Autodesk Inventor part; units mm, degrees
ref_plane "YZ Plane" through (0, 0, 0) normal (1, 0, 0) x (0, 1, 0)
ref_plane "XZ Plane" through (0, 0, 0) normal (0, 1, 0) x (-1, 0, 0)
ref_plane "XY Plane" through (0, 0, 0) normal (0, 0, 1) x (1, 0, 0)
sketch "Sketch1" plane through (0, 0, 0) normal (0, 0, 1) x (1, 0, 0)
  line L0 (58.4, 13.1) -> (-58.4, 13.1)
  line L1 (-58.4, 13.1) -> (-58.4, -13.1)
  line L2 (-58.4, -13.1) -> (58.4, -13.1)
  line L3 (58.4, -13.1) -> (58.4, 13.1)
  line L4 (58.4, 13.1) -> (-58.4, -13.1) construction
  line L5 (-58.4, 13.1) -> (58.4, -13.1) construction
  point P0 (0, 0)
  dimension "d0" = 116.8
  dimension "d1" = 26.2
extrude "Extrusion1" add sketch "Sketch1" along normal blind 11
sketch "Sketch2" plane through (58.4, -13.1, 0) normal (1, 0, 0) x (0, 0, -1)
  line L0 (0, 0) -> (0, 26.2)
  line L1 (0, 26.2) -> (-11, 26.2)
  line L2 (-11, 0) -> (-11, 26.2)
  line L3 (0, 0) -> (-11, 0)
  line L4 (-11, 26.2) -> (-11, 0)
  line L5 (-11, 26.2) -> (-5, 26.2)
  line L6 (-5, 26.2) -> (-5, 23.2)
  line L7 (-5, 23.2) -> (-11, 23.2)
  line L8 (-11, 23.2) -> (-11, 26.2)
  line L9 (-11, 23.2) -> (-8.4, 23.2)
  line L10 (-8.4, 23.2) -> (-8.4, 20.2)
  line L11 (-8.4, 20.2) -> (-11, 20.2)
  line L12 (-11, 20.2) -> (-11, 23.2)
  line L13 (-11, 26.2) -> (-5, 26.2)
  line L14 (-5, 26.2) -> (-5, 10.1)
  line L15 (-5, 10.1) -> (-11, 10.1)
  line L16 (-11, 10.1) -> (-11, 26.2)
  line L17 (-11, 10.1) -> (-5, 10.1)
  line L18 (-5, 10.1) -> (-5, 13.1)
  line L19 (-5, 13.1) -> (-11, 13.1)
  line L20 (-11, 13.1) -> (-11, 10.1)
  line L21 (-11, 13.1) -> (-8.4, 13.1)
  line L22 (-8.4, 13.1) -> (-8.4, 16.1)
  line L23 (-8.4, 16.1) -> (-11, 16.1)
  line L24 (-11, 16.1) -> (-11, 13.1)
  point P0 (0, 13.1)
  point P1 (-11, 16.1)
  point P2 (-11, 20.2)
  dimension "d4" = 6
  dimension "d5" = 3
  dimension "d6" = 2.6
  dimension "d7" = 3
  dimension "d8" = 16.1
  dimension "d9" = 3
  dimension "d10" = 2.6
  dimension "d11" = 3
extrude "Extrusion2" cut sketch "Sketch2" against normal blind 113.8 contours L14 L19 L22 L23 L2 L11 L10 L7
fillet "Fillet1" radius 2 5 edges at (58.4, 10.1, 11) (58.4, -5.05, 11) (-58.4, 0, 11) (58.4, 0, 0) (-58.4, 0, 0)
sketch "Sketch4" plane through (-56.4, -13.1, 0) normal (0, -1, 0) x (1, 0, 0)
  arc A0 (-2, 2) -> (0, 0) centre (0, 2) ccw
  line L0 (0, 0) -> (112.8, 0)
  arc A1 (112.8, 0) -> (114.8, 2) centre (112.8, 2) ccw
  line L1 (114.8, 2) -> (114.8, 9)
  arc A2 (114.8, 9) -> (112.8, 11) centre (112.8, 9) ccw
  line L2 (0, 11) -> (112.8, 11)
  arc A3 (0, 11) -> (-2, 9) centre (0, 9) ccw
  line L3 (-2, 2) -> (-2, 9)
  circle A4 centre (104.8, 5.5) radius 4.1
  circle A5 centre (97.8, 5.5) radius 2.15
  line L4 (97.8, 7.65) -> (101.3089, 7.65)
  line L5 (97.8, 3.35) -> (101.3089, 3.35)
  circle A6 centre (15, 5.5) radius 4.1
  circle A7 centre (8, 5.5) radius 2.15
  line L6 (8, 3.35) -> (11.5089, 3.35)
  line L7 (8, 7.65) -> (11.5089, 7.65)
  point P0 (56.4, 0)
  point P1 (114.8, 5.5)
  point P2 (12.2407, 8.5325)
  point P3 (8.4381, 3.3951)
  point P4 (11.1965, 3.9692)
  point P5 (-2, 5.5)
  dimension "d19" = 8.2
  dimension "d20" = 4.3
  dimension "d21" = 7
  dimension "d22" = 0
  dimension "d23" = 10
  dimension "d24" = 8.2
  dimension "d25" = 4.3
  dimension "d26" = 7
  dimension "d27" = 10
  dimension "d28" = 0
  dimension "d40" = 0
extrude "Extrusion4" cut sketch "Sketch4" against normal blind 5.2 contours A4 | A4 L5 A5 L4 | A5 | A6 | A6 L6 A7 L7 | A7
sketch "Sketch5" plane through (-56.4, -13.1, 0) normal (0, -1, 0) x (1, 0, 0)
  arc A0 (8, 7.65) -> (8, 3.35) centre (8, 5.5) ccw
  arc A1 (11.5089, 3.35) -> (11.5089, 7.65) centre (15, 5.5) ccw
  arc A2 (97.8, 7.65) -> (97.8, 3.35) centre (97.8, 5.5) ccw
  line L0 (97.8, 7.65) -> (101.3089, 7.65)
  arc A3 (101.3089, 3.35) -> (101.3089, 7.65) centre (104.8, 5.5) ccw
  line L1 (101.3089, 3.35) -> (97.8, 3.35)
  arc A4 (-2, 2) -> (0, 0) centre (0, 2) ccw
  line L2 (0, 0) -> (112.8, 0)
  arc A5 (112.8, 0) -> (114.8, 2) centre (112.8, 2) ccw
  line L3 (114.8, 2) -> (114.8, 9)
  arc A6 (114.8, 9) -> (112.8, 11) centre (112.8, 9) ccw
  line L4 (0, 11) -> (112.8, 11)
  arc A7 (0, 11) -> (-2, 9) centre (0, 9) ccw
  line L5 (-2, 2) -> (-2, 9)
  circle A8 centre (8, 5.5) radius 4.1
  line L6 (8, 9.6) -> (15, 9.6)
  line L7 (8, 1.4) -> (15, 1.4)
  arc A9 (11.5089, 3.35) -> (11.5089, 7.65) centre (15, 5.5) ccw
  circle A10 centre (97.8, 5.5) radius 4.1
  line L8 (97.8, 9.6) -> (104.8, 9.6)
  line L9 (104.8, 1.4) -> (97.8, 1.4)
  line L10 (8, 7.65) -> (11.5089, 7.65)
  line L11 (11.5089, 3.35) -> (8, 3.35)
  arc A11 (8, 7.65) -> (8, 3.35) centre (8, 5.5) ccw
  point P0 (56.4, 0)
  point P1 (19.1, 5.5)
  point P2 (19.1, 5.5)
  point P3 (5.85, 5.5)
  point P4 (95.65, 5.5)
  point P5 (12.4867, 2.2607)
  point P6 (12.4867, 8.7393)
  point P7 (96.275, 2.2698)
  point P8 (96.275, 8.7302)
  point P9 (5.85, 5.5)
  point P10 (101.2911, 7.65)
  point P11 (101.2911, 3.35)
  point P12 (11.4911, 3.35)
  point P13 (11.4911, 7.65)
  dimension "d32" = 8.2
  dimension "d33" = 0
  dimension "d35" = 8.2
  dimension "d36" = 0
  dimension "d42" = 0
  dimension "d43" = 0
extrude "Extrusion5" cut sketch "Sketch5" along normal blind 3.2 from surface at -5.2 contours L10 A8 L11 A0 | A0 L11 A8 L10 | A8 L6 A1 L10 | L11 A1 L7 A8 | L0 A10 L1 A2 | A2 L1 A10 L0 | A10 L8 A3 L0 | L1 A3 L9 A10
properties part number "module-slot" material "PC/ABS Plastic"
Geometry: final body of the model. Coordinates: model frame, mm. A direction names the side the tool comes from. Round coordinates to 2 decimals unless told otherwise and drop trailing zeros. Order: outer loops, then holes, each group sorted by start corner. A loop starts at its lowest first (then second) coordinate and runs counter-clockwise, first axis right, second up. Notation, with made-up numbers: (33.25, 9) - (61.25, 9) arc R21 cw to (61.25, 15) - close; hole circle Ø11 at (59, 23). An arc over 180 degrees is marked (long way). Write item = value, one per line. Start each with the question number.
Q1. Cut plane B-B on x = -8. Return the cut outline in (y, z), and give its area (3 significant figures).
Q2. Pull-direction query (Z, two-part tool) for faces 1 (the flat face through (58.4, -0.2, 5.5)), 2 (the cylindrical face through (-37.3, -11.1, 5.4)), 3 (the cylindrical face through (-57.8, -0.18, 10.43)); classes: +Z half, -Z half, draft (parallel to the pull), parting line (faces both ways), or undercut.
Q3. Ray query, line 1 (X direction, y = -10.8, z = 5.5); line 2 (Y direction, x = -49, z = 9.5); line 3 (Z direction, x = 35.5, y = 7.5). Return the intervals inside material, ascending. Write a range as from..to.
Q4. Access query for faces 4 (the cylindrical face through (-50.55, -12.11, 5.55)), 5 (the flat face through (-45, -7.9, 6)), 6 (the flat face through (2, 0, 7)). Directions: +Z, -Z, +X, -X, +Y, -Y. A direction counts if a zero-diameter tool reaches every point of the face in a straight line with its end or side. Return the directions, or none.
Q5. Cut plane A-A on y = 8.75. Return the cut outline in (x, z).
Outcome:
q1.outline = (-13.1, 0) - (13.1, 0) - (13.1, 11) - (7.1, 11) - (7.1, 8.4) - (10.1, 8.4) - (10.1, 5) - (0, 5) - (0, 8.4) - (3, 8.4) - (3, 11) - (-13.1, 11) - close
q1.area = 243 mm^2
q2.face_1 = draft
q2.face_2 = undercut
q2.face_3 = +Z half
q3.line_1 = -58.4..-52.5, -37.3..37.3, 52.5..58.4
q3.line_2 = -13.1..-11.1, -7.9..3, 7.1..13.1
q3.line_3 = 0..5, 8.4..11
q4.face_4 = -Y
q4.face_5 = none
q4.face_6 = +X
q5.outline = (-58.4, 2) arc R2 ccw to (-56.4, 0) - (56.4, 0) arc R2 ccw to (58.4, 2) - (58.4, 5) - (-55.4, 5) - (-55.4, 8.4) - (58.4, 8.4) - (58.4, 9) arc R2 ccw to (56.4, 11) - (-56.4, 11) arc R2 ccw to (-58.4, 9) - close
